Design review of the part built by this model. Coordinates are the model's own, in mm. Face numbers are marked on the shaded views. A direction names the side the tool comes from. Round coordinates to 2 decimals unless told otherwise and drop trailing zeros. Write each loop counter-clockwise with the first axis right and the second up, starting at its lowest first coordinate (ties: lowest second). Pieces come first, ordered by that corner, then holes. Notation, with made-up numbers: (58, 41.25) -> (117, 41.25) arc R24 cw to (117, 51.25) -> close; hole circle Ø7 at (36, -11.5). An arc over 180 degrees is marked (long way). One line per question, with ' | ' between items. Start each with the question number.
1) For probe 1 along Y at (x, z) = (18.5, 1.05); probe 2 along X at (y, z) = (-3, 12) (3 decimals), list the stretches that pass through material, from the lowest coordinate up.
2) Consider section A-A (y = 0). Give the boundary of the cut face in (x, z) (3 decimals).
3) For the marked faces 1, 2, 3 and 4, list the 3-axis set-ups (+Z, -Z, +X, -X, +Y, -Y) from which the entire face can be reached by the end or side of a thin tool; tool diameter is ignored.
4) Insertion check: pin 1 Ø2 at (x, z) = (-1.5, 9.5) entering from +Y; pin 2 Ø1.6 at (x, z) = (8.5, 12.5) entering from +Y; pin 3 Ø3 at (y, z) = (-3.5, 10.5) entering from -X. Each pin has a flat end and moves straight along its axis. Give the tip position at first contact, or say it passes through.
5) Consider section C-C (x = -1). Give the boundary of the cut face in (y, z), then the cut area to 3 significant figures.
6) Consider section D-D (y = -2). Give the boundary of the cut face in (x, z) (3 decimals).
7) Consider section B-B (z = 1.5). Give the boundary of the cut face in (x, y), then the cut area to 3 significant figures.
8) Mouldability with a two-part tool opening along X and no side actions: class the marked faces 5 and 6 as +X half, -X half, draft (parallel to the pull), parting line (faces both ways), or undercut.
```python
from build123d import *

# Parameters (mm, degrees)
F0_R     = 1.6
F1_DEPTH = 2
F2_W     = 29.5
F2_H     = 13
F3_DEPTH = 5.2
F4_W     = 29.5
F4_H     = 8.4
F5_DEPTH = 4.3
F6_W     = 16.3
F6_H     = 7.2
F6_W_2   = 7.5
F7_DEPTH = 2


with BuildPart() as f1:
    # F0 (on Top) → F1 (new body)
    with BuildSketch(Plane.XY):
        Polygon((14.75, 6.5), (-14.75, 6.5), (-14.75, 3.75), (-14.75, -3.75), (-14.75, -6.5), (14.75, -6.5), (14.75, -3.75), (14.75, 3.75), align=None)
        with BuildLine():
            Line((-14.75, -3.75), (-14.75, 3.75))
            Line((-14.75, 3.75), (-18.5, 3.75))
            ThreePointArc((-18.5, 3.75), (-22.25, 0), (-18.5, -3.75))
            Line((-18.5, -3.75), (-14.75, -3.75))
        make_face()
        with Locations((-18.5, 0)):
            Circle(F0_R, mode=Mode.SUBTRACT)
        with BuildLine():
            Line((18.5, 3.75), (14.75, 3.75))
            Line((14.75, 3.75), (14.75, -3.75))
            Line((14.75, -3.75), (18.5, -3.75))
            ThreePointArc((18.5, -3.75), (22.25, 0), (18.5, 3.75))
        make_face()
        with Locations((18.5, 0)):
            Circle(F0_R, mode=Mode.SUBTRACT)
    extrude(amount=F1_DEPTH)

    # F2 (on face) → F3 (join)
    with BuildSketch(Plane.XY.offset(2)):
        Rectangle(F2_W, F2_H)
    extrude(amount=F3_DEPTH)

    # F4 (on face) → F5 (join)
    with BuildSketch(Plane.XY.offset(7.2)):
        Rectangle(F4_W, F4_H)
    extrude(amount=F5_DEPTH)

    # F6 (on face) → F7 (join)
    with BuildSketch(Plane.XY.offset(11.5)):
        with Locations((5.825, 0)):
            Rectangle(F6_W, F6_H)
        with Locations((-10.225, 0)):
            Rectangle(F6_W_2, F6_H)
    extrude(amount=F7_DEPTH)


solid = f1.part
```
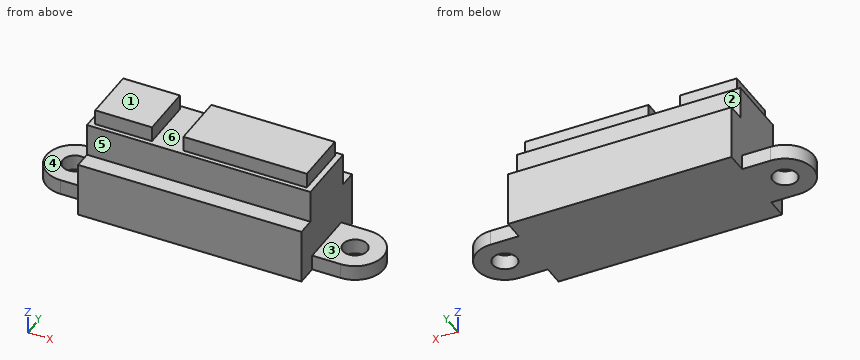
From the geometry:
1) probe 1: y = -3.75 to -1.6, 1.6 to 3.75 | probe 2: x = -13.975 to -6.475, -2.325 to 13.975
2) outline: (-22.25, 0) -> (-20.1, 0) -> (-20.1, 2) -> (-22.25, 2) -> close; (-16.9, 0) -> (16.9, 0) -> (16.9, 2) -> (14.75, 2) -> (14.75, 11.5) -> (13.975, 11.5) -> (13.975, 13.5) -> (-2.325, 13.5) -> (-2.325, 11.5) -> (-6.475, 11.5) -> (-6.475, 13.5) -> (-13.975, 13.5) -> (-13.975, 11.5) -> (-14.75, 11.5) -> (-14.75, 2) -> (-16.9, 2) -> close; (20.1, 0) -> (22.25, 0) -> (22.25, 2) -> (20.1, 2) -> close
3) face 1: +Z, +X, -X, +Y, -Y | face 2: +Z, +X, -X, +Y | face 3: +Z, +X, +Y, -Y | face 4: +Z, -X, +Y, -Y
4) pin 1: stops at y = 4.2 | pin 2: stops at y = 3.6 | pin 3: stops at x = -14.75
5) outline: (-6.5, 0) -> (6.5, 0) -> (6.5, 7.2) -> (4.2, 7.2) -> (4.2, 11.5) -> (3.6, 11.5) -> (3.6, 13.5) -> (-3.6, 13.5) -> (-3.6, 11.5) -> (-4.2, 11.5) -> (-4.2, 7.2) -> (-6.5, 7.2) -> close | area: 144 mm2
6) outline: (-21.672, 0) -> (21.672, 0) -> (21.672, 2) -> (14.75, 2) -> (14.75, 11.5) -> (13.975, 11.5) -> (13.975, 13.5) -> (-2.325, 13.5) -> (-2.325, 11.5) -> (-6.475, 11.5) -> (-6.475, 13.5) -> (-13.975, 13.5) -> (-13.975, 11.5) -> (-14.75, 11.5) -> (-14.75, 2) -> (-21.672, 2) -> close
7) outline: (-18.5, -3.75) -> (-14.75, -3.75) -> (-14.75, -6.5) -> (14.75, -6.5) -> (14.75, -3.75) -> (18.5, -3.75) arc R3.75 ccw to (18.5, 3.75) -> (14.75, 3.75) -> (14.75, 6.5) -> (-14.75, 6.5) -> (-14.75, 3.75) -> (-18.5, 3.75) arc R3.75 ccw to start; hole circle Ø3.2 at (-18.5, 0); hole circle Ø3.2 at (18.5, 0) | area: 468 mm2
8) face 5: draft | face 6: undercut
